from build123d import *

# Parameters (mm, degrees)
SKETCH2_R           = 13.75
BOSS_EXTRUDE1_DEPTH = 19.4


with BuildPart() as part:
    # Sketch2 → Boss-Extrude1 (new body)
    with BuildSketch(Plane.XY):
        with BuildLine():
            Line((-19.738634508, 20.767211648), (-19.738634508, -9.232788352))
            Line((-19.738634508, -9.232788352), (-3.735289218, -19.232788352))
            Line((-3.735289218, -19.232788352), (1.773741407, -19.232788352))
            ThreePointArc((1.773741407, -19.232788352), (17.434536233, -8.560097374), (17.984932853, 10.383605824))
            ThreePointArc((17.984932853, 10.383605824), (10.383605824, 17.984932853), (0, 20.767211648))
            Line((0, 20.767211648), (-19.738634508, 20.767211648))
        make_face()
        with Locations(Location((0, 0, 0), (0, 0, 180))):
            Circle(SKETCH2_R, mode=Mode.SUBTRACT)
    extrude(amount=BOSS_EXTRUDE1_DEPTH)


solid = part.part
CAD build for the part. Positions are in the model's coordinates, mm. Give positions to 0.01 mm unless a question says otherwise; leave off trailing zeros. Order: outer loops, then holes, each group sorted by start corner. A loop starts at its lowest first (then second) coordinate and runs counter-clockwise, first axis right, second up. Notation, with made-up numbers: (-34, 11.5) -> (2, 11.5) arc R21 ccw to (2, 40.5) -> close; hole circle Ø1 at (36.5, 21). An arc over 180 degrees is marked (long way). Return JSON: item names as keys, results as strings.
Q1. Saw through at D-D (x = -14.5). Write the cut outline in (y, z).
Working result:
{"outline": "(-12.51, 0) -> (20.77, 0) -> (20.77, 19.4) -> (-12.51, 19.4) -> close"}
Q2. Flat gauge pins, fed straight in: pin 1 (4 mm diameter, centred on x = -14, y = -6, fed in from -Z); pin 2 (6 mm diameter, centred on x = -10, z = 2.5, fed in from -Y); pin 3 (6 mm diameter, centred on x = 8, z = 3, fed in from -Y); pin 4 (4 mm diameter, centred on x = 6.5, z = 16.5, fed in from -Y). Where does each tip first touch, or does it go through?
Working result:
{"pin 1": "z = 0", "pin 2": "y = -17.19", "pin 3": "y = -18.56", "pin 4": "y = -18.7"}
Q3. Saw through at A-A (z = 17.5). Write the cut outline in (x, y).
Working result:
{"outline": "(-19.74, -9.23) -> (-3.74, -19.23) -> (1.77, -19.23) arc R20.85 ccw to (17.98, 10.38) arc R20.77 ccw to (0, 20.77) -> (-19.74, 20.77) -> close; hole circle Ø27.5 at (0, 0)"}
Q4. Mould opens along X. For faces 1 (the face through (0, 14, 0)), 2 (the face through (-6.34, 12.2, 9.56)), 3 (the face through (17.3, -8.8, 9.6)) say: pulls with the +X half, pulls with the -X half, needs draft (parallel to the pull), parting line crosses it, or undercut.
Working result:
{"face 1": "needs draft", "face 2": "undercut", "face 3": "pulls with the +X half"}
Q5. Saw through at B-B (x = 6). Write the cut outline in (y, z).
Working result:
{"outline": "(-18.24, 0) -> (-12.37, 0) -> (-12.37, 19.4) -> (-18.24, 19.4) -> close; (12.37, 0) -> (19.88, 0) -> (19.88, 19.4) -> (12.37, 19.4) -> close"}
Q6. Saw through at C-C (y = 13). Write the cut outline in (x, z).
Working result:
{"outline": "(-19.74, 0) -> (-4.48, 0) -> (-4.48, 19.4) -> (-19.74, 19.4) -> close; (4.48, 0) -> (16.19, 0) -> (16.19, 19.4) -> (4.48, 19.4) -> close"}
Q7. Drill centre lines: line 1 (Y direction, x = 0, z = 8.25); line 2 (X direction, y = -3, z = 15.25); line 3 (X direction, y = 10.5, z = 5.75). Where is each one in solid material? Low to high.
Working result:
{"line 1": "-19.23 to -13.75, 13.75 to 20.77", "line 2": "-19.74 to -13.42, 13.42 to 19.51", "line 3": "-19.74 to -8.88, 8.88 to 17.92"}
